Read the model definition and answer for the solid it produces. Units are mm, in the model's axes. A direction names the side the tool comes from. Round coordinates to 2 decimals unless told otherwise and drop trailing zeros. Order: outer loops, then holes, each group sorted by start corner. A loop starts at its lowest first (then second) coordinate and runs counter-clockwise, first axis right, second up. Notation, with made-up numbers: (72.25, 74) - (112.25, 74) arc R20 ccw to (112.25, 91) - close; hole circle Ø3 at (-19, 72). An arc over 180 degrees is marked (long way). One line per question, with ' | ' between items. Start each with the question number.
1) The part is cut by section A-A, the plane y = 24. Give the vertices of the cut face in (x, z).
2) The mould has two halves that part along Y. Classify faces 5 (the cylindrical face through (77, -3.1, 1.5)), 6 (the flat face through (39, 31, 3)), 7 (the cylindrical face through (76.923, 26.902, 1.521)), 8 (the cylindrical face through (87.034, -2.283, 1.479)): pulls with the +Y half, pulls with the -Y half, needs draft (parallel to the pull), parting line crosses it, or undercut.
3) Straight lines are drawn through the part: line 1 (Y direction, x = 51, z = 2.15); line 2 (Y direction, x = 17, z = 1.9); line 3 (Y direction, x = 20, z = 0.7). For each, find the intervals that lie inside material, in ascending order. Write a range as from..to.
4) The part is cut by section C-C, the plane x = 94. Give the vertices of the cut face in (y, z), plus the area to 3 significant figures.
5) Flat-ended cylindrical pins translate along their axes: pin 1 (0.9 mm diameter, centred on y = 10.5, z = 1, fed in from -X); pin 2 (1.5 mm diameter, centred on x = 35, z = 1.5, fed in from -Y); pin 3 (0.9 mm diameter, centred on x = 81, z = 1, fed in from +Y). Find the tip coordinate at first contact, or state that the pin passes through.
6) The part is cut by section D-D, the plane z = 0.75. Count the separate pieces of the cut face and the enclosed holes in it, plus the area to 3 significant figures.
7) For faces 1 (the flat face through (82, 30.402, 1)), 2 (the flat face through (82, -1.5, 1)), 3 (the flat face through (87.826, 18, 1)), 4 (the flat face through (47, 31, 0)), determine the directions among +Z, -Z, +X, -X, +Y, -Y from which every point of the face is accessible in a straight line to the end or side of a thin tool.
8) The part is cut by section B-B, the plane x = 45. Give the vertices of the cut face in (y, z).
from build123d import *

# Parameters (mm, degrees)
SKETCH1_R           = 1.25
SKETCH1_W           = 72.390227772
SKETCH1_H           = 28.901521269
BOSS_EXTRUDE1_DEPTH = 3
CHAMFER1_SIZE       = 1
SKETCH2_R           = 3.5
BOSS_EXTRUDE2_DEPTH = 3
CUT_EXTRUDE1_DEPTH  = 3


with BuildPart() as part:
    # Sketch1 → Boss-Extrude1 (new body)
    with BuildSketch(Plane.XY):
        with BuildLine():
            Line((6.173773471, 33.368208058), (-2.509184891, 52.727938114))
            ThreePointArc((-2.509184891, 52.727938114), (-1.316660917, 56.267635348), (2.304886114, 55.353323017))
            Line((2.304886114, 55.353323017), (91.695113886, 55.353323017))
            ThreePointArc((91.695113886, 55.353323017), (95.316660917, 56.267635348), (96.509184891, 52.727938114))
            Line((96.509184891, 52.727938114), (87.826226529, 33.368208058))
            Line((87.826226529, 33.368208058), (87.826226529, 1.466686789))
            ThreePointArc((87.826226529, 1.466686789), (86.983381771, -2.315616229), (83.195113886, -1.5))
            Line((83.195113886, -1.5), (10.804886114, -1.5))
            ThreePointArc((10.804886114, -1.5), (7.016618229, -2.315616229), (6.173773471, 1.466686789))
            Line((6.173773471, 1.466686789), (6.173773471, 33.368208058))
        make_face()
        with Locations((0, 53.853323017)):
            Circle(SKETCH1_R, mode=Mode.SUBTRACT)
        with Locations((8.5, 31.901521269)):
            Circle(SKETCH1_R, mode=Mode.SUBTRACT)
        with Locations((8.5, 0)):
            Circle(SKETCH1_R, mode=Mode.SUBTRACT)
        with Locations(Location((85.5, 0, 0), (0, 0, 180))):
            Circle(SKETCH1_R, mode=Mode.SUBTRACT)
        with Locations(Location((85.5, 31.901521269, 0), (0, 0, 180))):
            Circle(SKETCH1_R, mode=Mode.SUBTRACT)
        with Locations(Location((94, 53.853323017, 0), (0, 0, 180))):
            Circle(SKETCH1_R, mode=Mode.SUBTRACT)
        Polygon((10.804886114, 33.401521269), (2.304886114, 52.353323017), (91.695113886, 52.353323017), (83.195113886, 33.401521269), align=None, mode=Mode.SUBTRACT)
        with Locations((47, 15.950760635)):
            Rectangle(SKETCH1_W, SKETCH1_H, mode=Mode.SUBTRACT)
    extrude(amount=BOSS_EXTRUDE1_DEPTH)

    # Chamfer1
    chamfer1_edges = [part.edges().sort_by_distance(p)[0] for p in [
        (-1.25, 53.853323017, 3),
        (7.25, 31.901521269, 3),
        (7.25, 0, 3),
        (86.75, 0, 3),
        (86.75, 31.901521269, 3),
        (95.25, 53.853323017, 3),
    ]]
    chamfer(chamfer1_edges, length=CHAMFER1_SIZE)

    # Sketch2 → Boss-Extrude2 (add)
    with BuildSketch(Plane.XY.offset(3)):
        with Locations((17, 30.401521269)):
            Circle(SKETCH2_R)
        with Locations((17, 0.401521269)):
            Circle(SKETCH2_R)
        with Locations((77, 30.401521269)):
            Circle(SKETCH2_R)
        with Locations((77, 0.401521269)):
            Circle(SKETCH2_R)
    extrude(amount=-BOSS_EXTRUDE2_DEPTH)

    # Sketch2<3> → Cut-Extrude1 (cut)
    with BuildSketch(Plane.XY.offset(3)):
        with BuildLine():
            Line((15.978557649, 1.5), (18.021442351, 1.5))
            ThreePointArc((18.021442351, 1.5), (17, 1.901521269), (15.978557649, 1.5))
        make_face()
        with BuildLine():
            ThreePointArc((18.5, 0.401521269), (18.375166086, 1.000619121), (18.021442351, 1.5))
            Line((18.021442351, 1.5), (15.978557649, 1.5))
            ThreePointArc((15.978557649, 1.5), (16.400902148, -0.973644817), (18.5, 0.401521269))
        make_face()
        with BuildLine():
            Line((15.5, 30.401521269), (18.5, 30.401521269))
            ThreePointArc((18.5, 30.401521269), (17, 31.901521269), (15.5, 30.401521269))
        make_face()
        with BuildLine():
            ThreePointArc((15.5, 30.401521269), (17, 28.901521269), (18.5, 30.401521269))
            Line((18.5, 30.401521269), (15.5, 30.401521269))
        make_face()
        with BuildLine():
            Line((78.5, 30.401521269), (75.5, 30.401521269))
            ThreePointArc((75.5, 30.401521269), (77, 28.901521269), (78.5, 30.401521269))
        make_face()
        with BuildLine():
            ThreePointArc((78.5, 30.401521269), (77, 31.901521269), (75.5, 30.401521269))
            Line((75.5, 30.401521269), (78.5, 30.401521269))
        make_face()
        with BuildLine():
            Line((78.021442351, 1.5), (75.978557649, 1.5))
            ThreePointArc((75.978557649, 1.5), (76.400902148, -0.973644817), (78.5, 0.401521269))
            ThreePointArc((78.5, 0.401521269), (78.375166086, 1.000619121), (78.021442351, 1.5))
        make_face()
        with BuildLine():
            ThreePointArc((78.021442351, 1.5), (77, 1.901521269), (75.978557649, 1.5))
            Line((75.978557649, 1.5), (78.021442351, 1.5))
        make_face()
    extrude(amount=-CUT_EXTRUDE1_DEPTH, mode=Mode.SUBTRACT)


solid = part.part
Values:
1) outline: (6.17, 0) - (10.8, 0) - (10.8, 3) - (6.17, 3) - close; (83.2, 0) - (87.83, 0) - (87.83, 3) - (83.2, 3) - close
2) face 5: pulls with the -Y half | face 6: needs draft | face 7: undercut | face 8: undercut
3) line 1: y = -1.5..1.5, 30.4..33.4, 52.35..55.35 | line 2: y = -3.1..-1.1, 1.9..3.9, 26.9..28.9, 31.9..33.9, 52.35..55.35 | line 3: y = -1.5..2.2, 28.6..33.4, 52.35..55.35
4) outline: (47.13, 0) - (52.6, 0) - (52.6, 2) - (51.6, 3) - (47.13, 3) - close; (55.1, 0) - (56.6, 0) - (56.6, 3) - (56.1, 3) - (55.1, 2) - close | area: 19.9 mm^2
5) pin 1: stops at x = 6.17 | pin 2: stops at y = -1.5 | pin 3: stops at y = 55.35
6) separate pieces: 1 | enclosed holes: 12 | area: 1,270 mm^2
7) face 1: +Z, -Z | face 2: +Z, -Z, -Y | face 3: +Z, -Z, +X | face 4: -Z, +X, -X, +Y, -Y
8) outline: (-1.5, 0) - (1.5, 0) - (1.5, 3) - (-1.5, 3) - close; (30.4, 0) - (33.4, 0) - (33.4, 3) - (30.4, 3) - close; (52.35, 0) - (55.35, 0) - (55.35, 3) - (52.35, 3) - close
